Can you work these out from the drawing? Everything is in mm from the part's minimum corner. Coordinates: 2 decimals unless noted, no trailing zeros. Write each loop counter-clockwise with the first axis right and the second up, starting at its lowest first coordinate (ties: lowest second). Pieces come first, ordered by that corner, then holes. Notation, with made-up numbers: (13.5, 74.5) -> (72.5, 74.5) arc R29 cw to (72.5, 96.5) -> close; hole circle Ø3 at (76.25, -14.5). An arc over 180 degrees is marked (long way). Use a Markdown table: item, result. Add a question column.
Item 1: If I drill on line 1 along X through (y, z) = (26, 0.8); line 2 along Y through (x, z) = (14.75, 0.9), over which ranges is the centre line in solid material (lowest first)? Write a range as from..to.
Item 2: Imagine slicing it at B-B, the plane z = 0.85. Write out the boundary of the cut face in (x, y), and give its area (3 significant figures).
Item 3: Imagine slicing it at A-A, the plane y = 15. Write out the boundary of the cut face in (x, z), and give its area (3 significant figures).
Item 4: Imagine slicing it at D-D, the plane x = 3.25. Write out the boundary of the cut face in (y, z), and give its area (3 significant figures).
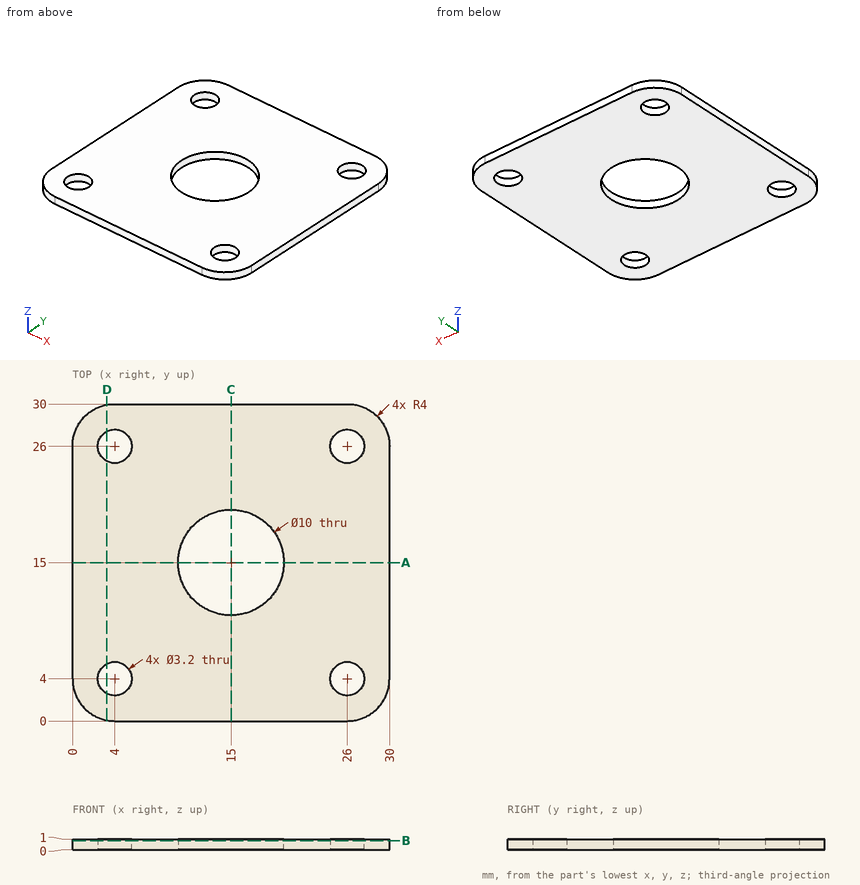
Ans:
| question | item | result |
|---|---|---|
| 1 | line 1 | x = 0..2.4, 5.6..24.4, 27.6..30 |
| 1 | line 2 | y = 0..10.01, 19.99..30 |
| 2 | outline | (0, 4) arc R4 ccw to (4, 0) -> (26, 0) arc R4 ccw to (30, 4) -> (30, 26) arc R4 ccw to (26, 30) -> (4, 30) arc R4 ccw to (0, 26) -> close; hole circle Ø3.2 at (4, 4); hole circle Ø3.2 at (4, 26); hole circle Ø10 at (15, 15); hole circle Ø3.2 at (26, 4); hole circle Ø3.2 at (26, 26) |
| 2 | area | 776 mm^2 |
| 3 | outline | (0, 0) -> (10, 0) -> (10, 1) -> (0, 1) -> close; (20, 0) -> (30, 0) -> (30, 1) -> (20, 1) -> close |
| 3 | area | 20.0 mm^2 |
| 4 | outline | (0.07, 0) -> (2.59, 0) -> (2.59, 1) -> (0.07, 1) -> close; (5.41, 0) -> (24.59, 0) -> (24.59, 1) -> (5.41, 1) -> close; (27.41, 0) -> (29.93, 0) -> (29.93, 1) -> (27.41, 1) -> close |
| 4 | area | 24.2 mm^2 |
